Source: CAD feature listing. Evaluate the final solid. Frame: model axes, mm. A direction names the side the tool comes from. Give positions to 0.01 mm unless a question says otherwise; leave off trailing zeros. Order: outer loops, then holes, each group sorted by start corner. A loop starts at its lowest first (then second) coordinate and runs counter-clockwise, first axis right, second up.
Autodesk Inventor part; units mm, degrees
ref_plane "YZ Plane" through (0, 0, 0) normal (1, 0, 0) x (0, 1, 0)
ref_plane "XZ Plane" through (0, 0, 0) normal (0, 1, 0) x (-1, 0, 0)
ref_plane "XY Plane" through (0, 0, 0) normal (0, 0, 1) x (1, 0, 0)
sketch "Sketch2" plane through (0, 0, 0) normal (0, 0, 1) x (1, 0, 0)
  line L0 (0, 0) -> (0, 6)
  line L1 (0, 6) -> (-6, 6)
  line L2 (-6, 6) -> (6, 6)
  line L3 (6, 6) -> (6, -16.5)
  line L4 (6, -16.5) -> (-6, -16.5)
  line L5 (-6, -16.5) -> (-6, 6)
  circle A0 centre (0, 0) radius 40
  line L6 (6.3, 6.3) -> (-6.3, 6.3)
  line L7 (-6.3, 6.3) -> (-6.3, -16.8)
  line L8 (-6.3, -16.8) -> (6.3, -16.8)
  line L9 (6.3, -16.8) -> (6.3, 6.3)
  dimension "d15" = 6
  dimension "d16" = 6
  dimension "d17" = 12
  dimension "d18" = 22.5
  dimension "d19" = 80
  dimension "d20" = 0.3
extrude "Extrusion4" add sketch "Sketch2" along normal blind 6.5 contours A0
sketch "Sketch3" plane through (0, 0, 6.5) normal (0, 0, 1) x (1, 0, 0)
  line L0 (-6.3, 6.3) -> (6.3, 6.3)
  line L1 (0, 6.3) -> (0, 8.25)
  circle A0 centre (0, 8.25) radius 0.5
  line L2 (6.3, -16.8) -> (-6.3, -16.8)
  line L3 (0, -16.8) -> (0, -18.75)
  circle A1 centre (0, -18.75) radius 0.5
  point P0 (0, 0)
  dimension "d23" = 1.95
  dimension "d24" = 1
  dimension "d25" = 1.95
  dimension "d26" = 1
extrude "Extrusion5" cut sketch "Sketch3" against normal blind 5.5
sketch "Sketch5" plane through (0, 0, 6.5) normal (0, 0, 1) x (1, 0, 0)
  circle A0 centre (0, 0) radius 40
sketch "Sketch6" plane through (0, 0, 6.5) normal (0, 0, 1) x (1, 0, 0)
  line L0 (0, 0) -> (0, -42)
  line L1 (0, -42) -> (0, 42)
  circle A0 centre (0, 42) radius 2.5
  circle A1 centre (0, 42) radius 6
  circle A2 centre (0, -42) radius 2.5
  circle A3 centre (0, -42) radius 6
  dimension "d46" = 42
  dimension "d47" = 84
  dimension "d48" = 5
  dimension "d49" = 12
  dimension "d50" = 5
  dimension "d51" = 12
extrude "Extrusion9" add sketch "Sketch6" against normal blind 6.5 contours A2 | A3 | A0 | A1
extrude "Extrusion10" cut sketch "Sketch6" against normal blind 6.5 contours A2 | A0
fillet "Fillet2" radius 12 4 edges at (5.5074, -39.619, 3.25) (-5.5074, -39.619, 3.25) (5.5074, 39.619, 3.25) (-5.5074, 39.619, 3.25)
sketch "Sketch8" plane through (0, 0, 6.5) normal (0, 0, 1) x (1, 0, 0)
  circle A0 centre (0, 0) radius 26.3
  dimension "d58" = 52.6
extrude "Extrusion11" cut sketch "Sketch8" against normal blind 1.3
sketch "Sketch9" plane through (0, 0, 6.5) normal (0, 0, 1) x (1, 0, 0)
  arc A0 (-29.3, 0) -> (29.3, 0) centre (0, 0) ccw
  arc A1 (-31.3, 0) -> (31.0101, -4.25) centre (0, 0) ccw
  line L0 (29.3, 0) -> (29.3, 4.25)
  line L1 (29.3, 4.25) -> (32.8, 4.25)
  line L2 (32.8, 4.25) -> (32.8, -4.25)
  line L3 (32.8, -4.25) -> (31.0101, -4.25)
  line L4 (-31.3, 0) -> (-29.3, 0)
  dimension "d61" = 29.3
  dimension "d62" = 31.3
  dimension "d63" = 4.25
  dimension "d64" = 3.5
  dimension "d65" = 8.5
extrude "Extrusion12" cut sketch "Sketch9" against normal blind 10
properties part number "Onderste plaat bevestiging axiale lager" material "S235"
1) Reachability of faces 1 (the face through (9, 25, 6.5)), 2 (the face through (31, 4.25, 3)), 3 (the face through (11, 0, 5.2)) from +Z, -Z, +X, -X, +Y, -Y: full face, straight path, thin tool, end or side. Return the list, or none.
Checks:
face 1: +Z, +X, -X, +Y, -Y
face 2: +Z, -Z
face 3: +Z
2) First-contact query: pin 1 Ø0.5 at (x, z) = (32, 3) entering from +Y; pin 2 Ø0.8 at (x, y) = (0, 8) entering from +Z; pin 3 Ø2 at (y, z) = (-17.5, 3) entering from -X; pin 4 Ø2 at (x, y) = (-12.5, -16.5) entering from -Z. Flat tips, straight axial feed; report the tip coordinate or a pass-through.
Checks:
pin 1: stops at y = 24.33
pin 2: stops at z = 5.2
pin 3: stops at x = -36.44
pin 4: stops at z = 0
3) Ray query, L1, parallel to Y at x = 0, z = 5.25; L2, parallel to Y at x = -15, z = 5.75; L3, parallel to Y at x = 3, z = 2. Return the intervals inside material, ascending.
Checks:
L1: y = -48 to -44.5, -39.5 to -31.3, -29.3 to -26.3, 26.3 to 39.5, 44.5 to 48
L2: y = -37.08 to -27.47, -25.17 to -21.6, 21.6 to 37.08
L3: y = -47.2 to -31.16, -29.15 to -16.8, 6.3 to 47.2
4) Section query A-A on x = -14. Output: boundary loops of the cut face in (y, z).
Checks:
outline: (-37.47, 0) - (-27.99, 0) - (-27.99, 6.5) - (-37.47, 6.5) - close; (-25.74, 0) - (37.47, 0) - (37.47, 6.5) - (22.26, 6.5) - (22.26, 5.2) - (-22.26, 5.2) - (-22.26, 6.5) - (-25.74, 6.5) - close
5) Section query B-B on y = 2.5. Output: boundary loops of the cut face in (x, z).
Checks:
outline: (-39.92, 0) - (-6.3, 0) - (-6.3, 5.2) - (-26.18, 5.2) - (-26.18, 6.5) - (-39.92, 6.5) - close; (6.3, 0) - (29.3, 0) - (29.3, 6.5) - (26.18, 6.5) - (26.18, 5.2) - (6.3, 5.2) - close; (32.8, 0) - (39.92, 0) - (39.92, 6.5) - (32.8, 6.5) - close
6) Pull-direction query (X, two-part tool) for faces 4 (the face through (-26.275, 1.156, 5.859)), 5 (the face through (-39.994, -0.699, 3.204)), 6 (the face through (0, 48, 3)); classes: +X half, -X half, draft (parallel to the pull), parting line (faces both ways), or undercut.
Checks:
face 4: undercut
face 5: -X half
face 6: parting line
7) Section query C-C on y = -36. Output: boundary loops of the cut face in (x, z).
Checks:
outline: (-17.44, 0) - (17.44, 0) - (17.44, 6.5) - (-17.44, 6.5) - close
